Check sheet for the modelled part. Datum: model origin and axes. Units: mm. Round coordinates to 2 decimals unless told otherwise and drop trailing zeros. Order: outer loops, then holes, each group sorted by start corner. A loop starts at its lowest first (then second) coordinate and runs counter-clockwise, first axis right, second up.
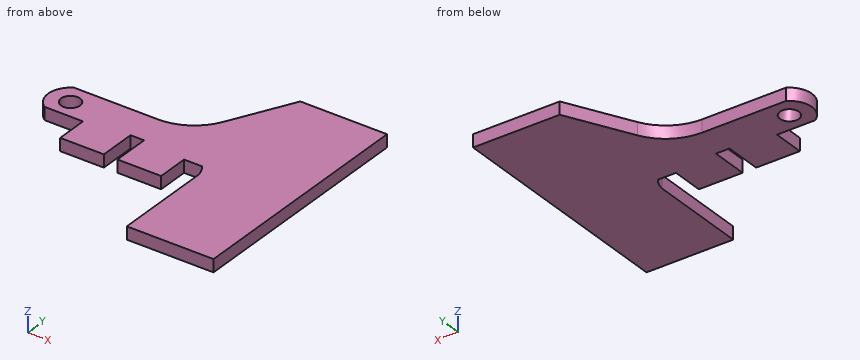
```python
from build123d import *

# Parameters (mm, degrees)
COPYSKETCH004_R = 3.02
PAD_DEPTH       = 2


with BuildPart() as part:
    # CopySketch004 → Pad (new body, symmetric)
    with BuildSketch(Plane.XY):
        with BuildLine():
            Line((-27.534542, 12.08528), (-1.01073, 12.08528))
            ThreePointArc((-1.01073, 12.08528), (7.323138, 14.431249), (13.209413, 20.780161))
            Line((13.209413, 20.780161), (23.383837, 40.65183))
            Line((23.383837, 40.65183), (50.86044, 40.65183))
            Line((50.86044, 40.65183), (50.86044, 0))
            Line((50.86044, -35.221027), (50.86044, 0))
            Line((23.383837, -35.221027), (50.86044, -35.221027))
            Line((23.401691, -4.060687), (23.383837, -35.221027))
            ThreePointArc((23.401691, -4.060687), (22.843077, -1.909417), (21.705474, 0))
            Line((16, 0), (21.705474, 0))
            Line((16, -10), (16, 0))
            Line((2.15, -10), (16, -10))
            Line((2.15, 1.647389), (2.15, -10))
            Line((-2.15, 1.647389), (2.15, 1.647389))
            Line((-2.15, -10), (-2.15, 1.647389))
            Line((-16, -10), (-2.15, -10))
            Line((-16, 0), (-16, -10))
            Line((-16, 0), (-28.183644, 0))
            ThreePointArc((-27.534542, 12.08528), (-31.259646, 6.225284), (-28.183644, 0))
        make_face()
        with Locations((-24.190611, 5.845606)):
            Circle(COPYSKETCH004_R, mode=Mode.SUBTRACT)
    extrude(amount=PAD_DEPTH, both=True)


solid = part.part
```
Item 1: Sectioned sample at B-B (y = -1). Record the cut outline in (x, z).
Answer:
outline: (-16, -2) - (-2.15, -2) - (-2.15, 2) - (-16, 2) - close; (2.15, -2) - (16, -2) - (16, 2) - (2.15, 2) - close; (22.39, -2) - (50.86, -2) - (50.86, 2) - (22.39, 2) - close
Item 2: Scan lines: line 1 along X through (y, z) = (-4, -0.95); line 2 along X through (y, z) = (-15, -0.6); line 3 along Y through (x, z) = (-19.5, -0.85). Record each from-to range of solid material in increasing order.
Answer:
line 1: x = -16 to -2.15, 2.15 to 16, 23.39 to 50.86
line 2: x = 23.4 to 50.86
line 3: y = 0 to 12.09
Item 3: Sectioned sample at A-A (y = 7). Record the cut outline in (x, z).
Answer:
outline: (-31.18, -2) - (-26.98, -2) - (-26.98, 2) - (-31.18, 2) - close; (-21.4, -2) - (50.86, -2) - (50.86, 2) - (-21.4, 2) - close
Item 4: Sectioned sample at D-D (x = -5). Record the cut outline in (y, z).
Answer:
outline: (-10, -2) - (12.09, -2) - (12.09, 2) - (-10, 2) - close
Item 5: Sectioned sample at C-C (z = -0.75). Record the cut outline in (x, y).
Answer:
outline: (-28.18, 0) - (-16, 0) - (-16, -10) - (-2.15, -10) - (-2.15, 1.65) - (2.15, 1.65) - (2.15, -10) - (16, -10) - (16, 0) - (21.71, 0) arc R7.87 cw to (23.4, -4.06) - (23.38, -35.22) - (50.86, -35.22) - (50.86, 40.65) - (23.38, 40.65) - (13.21, 20.78) arc R15.98 cw to (-1.01, 12.09) - (-27.53, 12.09) arc R7.08 ccw to start; hole circle Ø6.04 at (-24.19, 5.85)
Item 6: Go/stop test with flat-tipped pins: P1, Ø1.2, axis at x = -23.5, z = 0, coming from the -Y side; P2, Ø1.2, axis at x = -9, z = 1, coming from the -Y side; P3, Ø1.2, axis at y = -6.5, z = 1, coming from the -X side. Record where each tip stops, or that it passes through.
Answer:
P1: stops at y = 0
P2: stops at y = -10
P3: stops at x = -16
